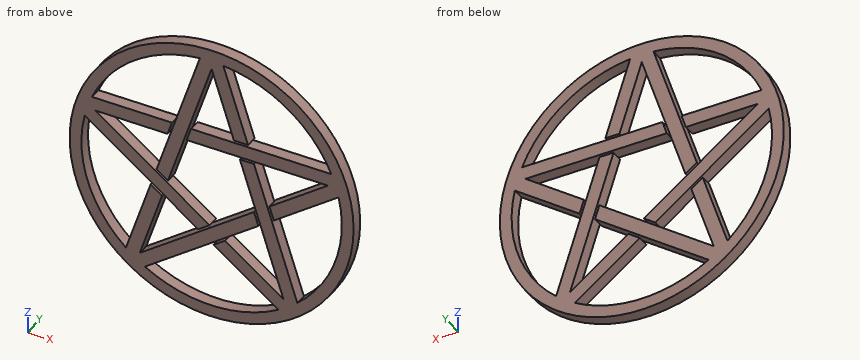
from build123d import *

# Parameters (mm, degrees)
F0_R     = 76.541025
F1_DEPTH = 6.35


with BuildPart() as f1:
    # F0 (on Front) → F1 (new body)
    with BuildSketch(Plane.XZ):
        Circle(F0_R)
        with BuildLine():
            ThreePointArc((-64.53644, 27.601229), (-41.257249, 56.785732), (-6.307472, 69.907051))
            Line((-6.307472, 69.907051), (-29.685655, -2.043597))
            Line((-29.685655, -2.043597), (-23.536186, -6.511448))
            Line((-23.536186, -6.511448), (0, 65.925484))
            Line((0, 65.925484), (12.039657, 28.871229))
            Line((12.039657, 28.871229), (19.640819, 28.871229))
            Line((19.640819, 28.871229), (6.307472, 69.907051))
            ThreePointArc((6.307472, 69.907051), (41.257249, 56.785732), (64.53644, 27.601229))
            Line((64.53644, 27.601229), (-11.116948, 27.601229))
            Line((-11.116948, 27.601229), (-13.465836, 20.372095))
            Line((-13.465836, 20.372095), (62.698861, 20.372095))
            Line((62.698861, 20.372095), (31.17863, -2.528694))
            Line((31.17863, -2.528694), (33.527518, -9.757828))
            Line((33.527518, -9.757828), (68.434673, 15.603704))
            ThreePointArc((68.434673, 15.603704), (66.755632, -21.69022), (46.193186, -52.848553))
            Line((46.193186, -52.848553), (22.815003, 19.102095))
            Line((22.815003, 19.102095), (15.213841, 19.102095))
            Line((15.213841, 19.102095), (38.750027, -53.334837))
            Line((38.750027, -53.334837), (7.229796, -30.434048))
            Line((7.229796, -30.434048), (1.080327, -34.901899))
            Line((1.080327, -34.901899), (35.987481, -60.263432))
            ThreePointArc((35.987481, -60.263432), (0, -70.191025), (-35.987481, -60.263432))
            Line((-35.987481, -60.263432), (25.217396, -15.795485))
            Line((25.217396, -15.795485), (22.868507, -8.566351))
            Line((22.868507, -8.566351), (-38.750027, -53.334837))
            Line((-38.750027, -53.334837), (-26.71037, -16.280582))
            Line((-26.71037, -16.280582), (-32.859839, -11.812731))
            Line((-32.859839, -11.812731), (-46.193186, -52.848553))
            ThreePointArc((-46.193186, -52.848553), (-66.755632, -21.69022), (-68.434673, 15.603704))
            Line((-68.434673, 15.603704), (-7.229796, -28.864242))
            Line((-7.229796, -28.864242), (-1.080327, -24.396391))
            Line((-1.080327, -24.396391), (-62.698861, 20.372095))
            Line((-62.698861, 20.372095), (-23.737712, 20.372095))
            Line((-23.737712, 20.372095), (-21.388824, 27.601229))
            Line((-21.388824, 27.601229), (-64.53644, 27.601229))
        make_face(mode=Mode.SUBTRACT)
    extrude(amount=F1_DEPTH)


solid = f1.part
Verification items for the finished model (mm, model axes). Coordinates: 2 decimals unless noted, no trailing zeros. Order: outer loops, then holes, each group sorted by start corner. A loop starts at its lowest first (then second) coordinate and runs counter-clockwise, first axis right, second up. Notation, with made-up numbers: M -31,-20 L -20,-20 A19 ccw -20,-13 Z; hole C -17,17 d6. An arc over 180 degrees is marked long. One line per item, written item: value. Start each with the question number.
Item 1: Gauge pin test, flat ends, axial feed: pin 1 (1.9 mm diameter, centred on x = 16.5, y = -3, fed in from -Z); pin 2 (1.9 mm diameter, centred on x = 31.5, y = -4.5, fed in from -Z); pin 3 (1 mm diameter, centred on x = 35.5, y = -2.5, fed in from -Z); pin 4 (6 mm diameter, centred on x = 58, z = -28.5, fed in from +Y). Record the tip position at first contact, or that the pin passes through.
Item 2: Sectioned sample at B-B (x = -42). Enter the section's corners in (y, z).
Item 3: Scan lines: probe 1 along X at (y, z) = (-0.5, 51); probe 2 along X at (y, z) = (-2.75, 60) (3 decimals); probe 3 along X at (y, z) = (-4.75, 26.5). Record each from-to range of solid material in increasing order.
Item 4: Sectioned sample at C-C (z = 0). Enter the section's corners in (x, y).
Item 5: Sectioned sample at A-A (z = 49.5). Enter the section's corners in (x, y), then the cut area to 3 significant figures.
Conclusion:
1. pin 1: stops at z = -74.94
1. pin 2: stops at z = -70.18
1. pin 3: stops at z = -68.07
1. pin 4: passes through
2. outline: M -6.35,-63.99 L 0,-63.99 L 0,-39.94 L -6.35,-39.94 Z; M -6.35,-3.6 L 0,-3.6 L 0,5.33 L -6.35,5.33 Z; M -6.35,20.37 L 0,20.37 L 0,27.6 L -6.35,27.6 Z; M -6.35,56.24 L 0,56.24 L 0,63.99 L -6.35,63.99 Z
3. probe 1: x = -57.07 to -48.23, -12.45 to -4.85, 4.85 to 12.45, 48.23 to 57.07
3. probe 2: x = -47.524 to -36.425, -9.526 to -1.925, 1.925 to 9.526, 36.425 to 47.524
3. probe 3: x = -71.81 to -21.75, -20.41 to -12.81, -11.47 to 71.81
4. outline: M -76.54,-6.35 L -70.19,-6.35 L -70.19,0 L -76.54,0 Z; M -46.96,-6.35 L -34.66,-6.35 L -34.66,0 L -46.96,0 Z; M -29.02,-6.35 L -21.42,-6.35 L -21.42,0 L -29.02,0 Z; M 21.42,-6.35 L 29.02,-6.35 L 29.02,0 L 21.42,0 Z; M 34.66,-6.35 L 46.96,-6.35 L 46.96,0 L 34.66,0 Z; M 70.19,-6.35 L 76.54,-6.35 L 76.54,0 L 70.19,0 Z
5. outline: M -58.38,-6.35 L -49.76,-6.35 L -49.76,0 L -58.38,0 Z; M -12.94,-6.35 L -5.34,-6.35 L -5.34,0 L -12.94,0 Z; M 5.34,-6.35 L 12.94,-6.35 L 12.94,0 L 5.34,0 Z; M 49.76,-6.35 L 58.38,-6.35 L 58.38,0 L 49.76,0 Z
5. area: 206 mm^2
